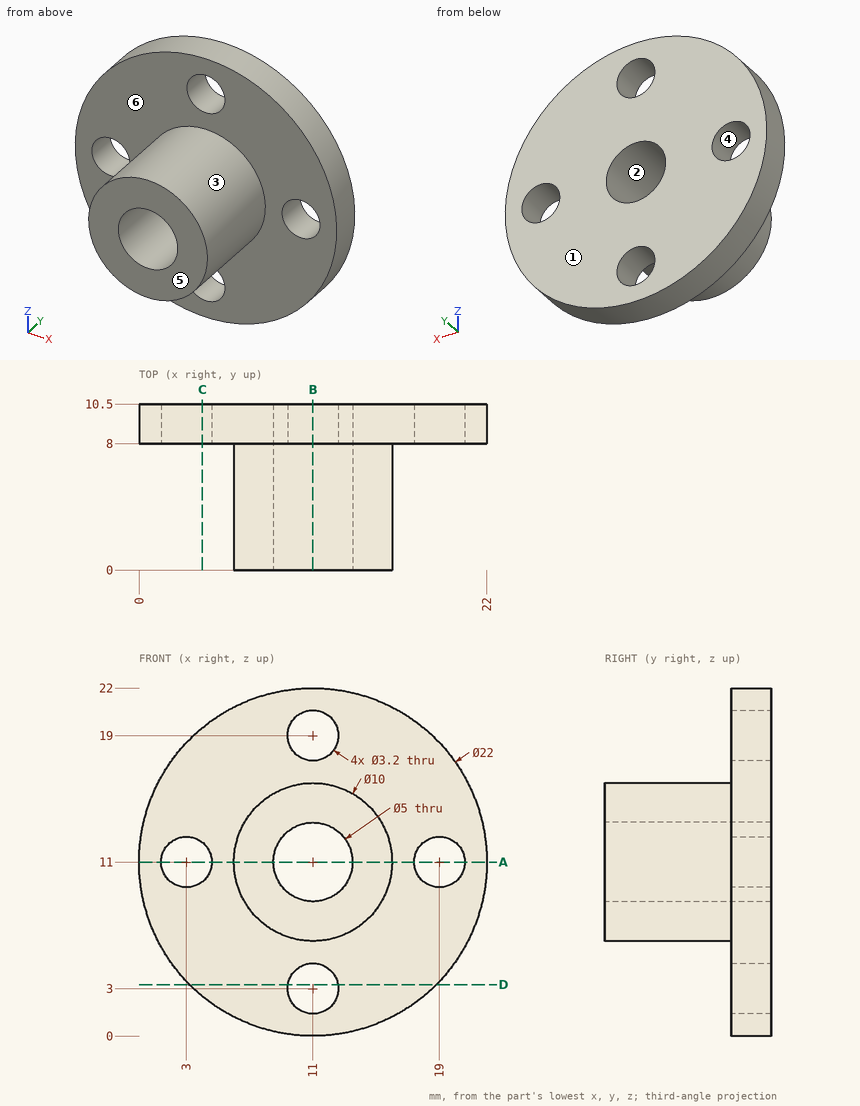
For this review, use the dimensioned drawing (mm, ordinates from the lowest corner) and the shaded views. A direction names the side the tool comes from. Coordinates: 2 decimals unless noted, no trailing zeros. Loops run counter-clockwise (first coordinate to the right, second up) from the corner with the lowest first, then second, coordinate; pieces in that order, holes last. Notation, with made-up numbers: (-32.75, -37) - (-23.75, -37) arc R14 ccw to (-23.75, -15) - close; hole circle Ø7 at (75.5, -5.5). An arc over 180 degrees is marked (long way). Use CSV: the item, a comma, the result in double quotes. Start each with the question number.
1) Consider section B-B on x = 11. Write out the cut boundary in (y, z).
2) Consider section C-C on x = 4. Write out the cut boundary in (y, z).
3) The part is to be moulded in two halves that separate along Z. For the marked faces 1, 2, 3 and 4, say which applies: +Z half, -Z half, draft (parallel to the pull), parting line (faces both ways), or undercut.
4) Consider section D-D on z = 3.25. Write out the cut boundary in (x, y), then the cut area to 3 significant figures.
5) Wall thickness on L1, parallel to X at y = 9.7, z = 11; L2, parallel to Y at x = 17, z = 12.25; L3, parallel to Z at x = 11.5, y = 4.5: over which ranges is each line inside the solid? List them lowest first. Write a range as from..to.
6) Tool access review of the marked faces 5 and 6: name each direction out of +Z, -Z, +X, -X, +Y, -Y from which nothing blocks a thin tool from reaching the whole face with its end or side.
7) Consider section A-A on z = 11. Write out the cut boundary in (x, y).
8) For pin 1 Ø2 at (y, z) = (5.5, 10) entering from -X; pin 2 Ø11 at (x, z) = (8, 13) entering from -Y; pin 3 Ø5 at (x, z) = (3, 11) entering from -Y; pin 4 Ø1.5 at (y, z) = (8.5, 16) entering from +X, all flat-tipped, find the tip position at first contact; note any pin that passes through.
Geometry says:
1,outline,"(0, 6) - (8, 6) - (8, 4.6) - (10.5, 4.6) - (10.5, 8.5) - (0, 8.5) - close; (0, 13.5) - (10.5, 13.5) - (10.5, 17.4) - (8, 17.4) - (8, 16) - (0, 16) - close; (8, 0) - (10.5, 0) - (10.5, 1.4) - (8, 1.4) - close; (8, 20.6) - (10.5, 20.6) - (10.5, 22) - (8, 22) - close"
2,outline,"(8, 2.51) - (10.5, 2.51) - (10.5, 9.75) - (8, 9.75) - close; (8, 12.25) - (10.5, 12.25) - (10.5, 19.49) - (8, 19.49) - close"
3,face 1,"draft"
3,face 2,"undercut"
3,face 3,"parting line"
3,face 4,"undercut"
4,outline,"(3.19, 8) - (9.42, 8) - (9.42, 10.5) - (3.19, 10.5) - close; (12.58, 8) - (18.81, 8) - (18.81, 10.5) - (12.58, 10.5) - close"
4,area,"31.1 mm^2"
5,L1,"0..1.4, 4.6..8.5, 13.5..17.4, 20.6..22"
5,L2,"8..10.5"
5,L3,"6.03..8.55, 13.45..15.97"
6,face 5,"+Z, -Z, +X, -X, -Y"
6,face 6,"-Y"
7,outline,"(0, 8) - (1.4, 8) - (1.4, 10.5) - (0, 10.5) - close; (4.6, 8) - (6, 8) - (6, 0) - (8.5, 0) - (8.5, 10.5) - (4.6, 10.5) - close; (13.5, 0) - (16, 0) - (16, 8) - (17.4, 8) - (17.4, 10.5) - (13.5, 10.5) - close; (20.6, 8) - (22, 8) - (22, 10.5) - (20.6, 10.5) - close"
8,pin 1,"x = 6"
8,pin 2,"y = 0"
8,pin 3,"y = 8"
8,pin 4,"x = 21.15"
